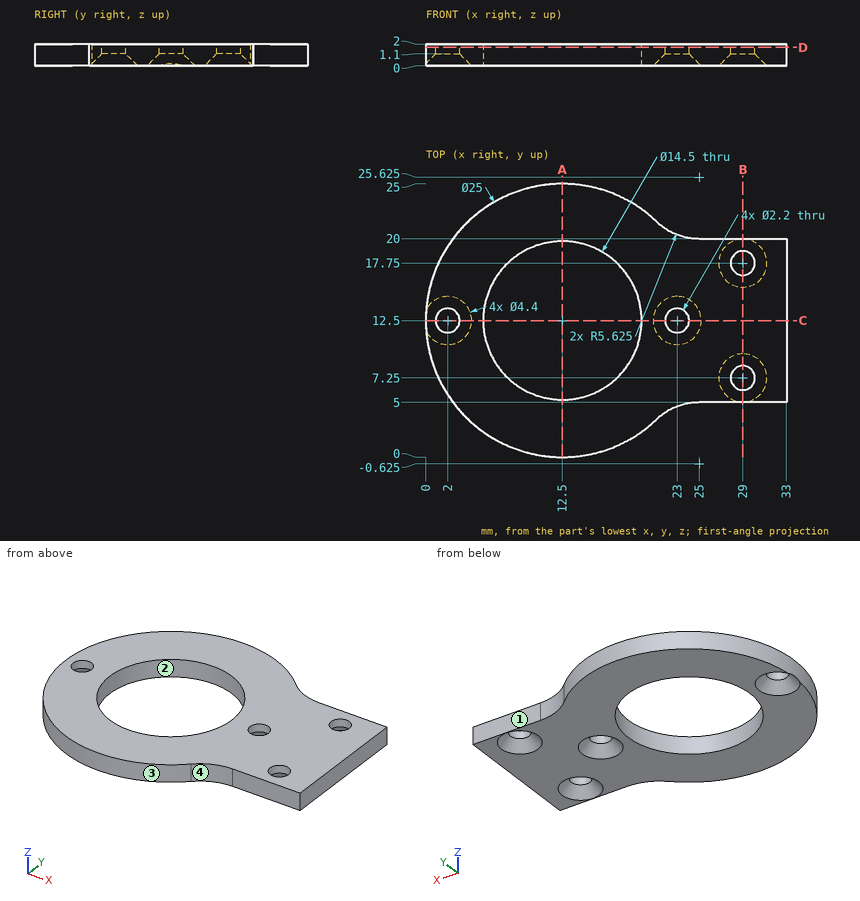
Geometry check sheet. Reference: drawing and pictorial views, mm from the part's lowest x, y, z. Round coordinates to 2 decimals unless told otherwise and drop trailing zeros. Order: outer loops, then holes, each group sorted by start corner. A loop starts at its lowest first (then second) coordinate and runs counter-clockwise, first axis right, second up. Notation, with made-up numbers: (20.5, 57.5) -> (49.5, 57.5) arc R36 ccw to (49.5, 92.5) -> close; hole circle Ø9 at (6, -2). An arc over 180 degrees is marked (long way). One line per item, written item: value. Start each with the question number.
Q1. Cross-section at C-C (y = 12.5). Record the boundary of the cut face in (x, z).
Q2. Gauge pin test, flat ends, axial feed: pin 1 Ø0.6 at (x, z) = (28.5, 1) entering from +Y; pin 2 Ø1.3 at (x, y) = (23, 12.5) entering from +Z; pin 3 Ø3.5 at (x, y) = (29, 7.25) entering from -Z. Record the tip position at first contact, or that the pin passes through.
Q3. Cross-section at A-A (x = 12.5). Record the boundary of the cut face in (y, z), and give its area (3 significant figures).
Q4. Cross-section at D-D (z = 1.7). Record the boundary of the cut face in (x, y) (3 decimals), and give its area (3 significant figures).
Q5. Mould release check, pull along Y, two halves, no side actions. Record for the marked faces 1, 2, 3 and 4: pulls with the +Y half, pulls with the -Y half, needs draft (parallel to the pull), parting line crosses it, or undercut.
Q6. Cross-section at B-B (x = 29). Record the boundary of the cut face in (y, z), and give its area (3 significant figures).
Q7. Thickness scan on line 1 (Y direction, x = 12.5, z = 1.4); line 2 (X direction, y = 18.5, z = 0.4); line 3 (X direction, y = 6.25, z = 1.7) (1 decimal). Record the ranges inside material, lowest first.
Completed:
1. outline: (0, 0.2) -> (0.9, 1.1) -> (0.9, 2) -> (0, 2) -> close; (3.1, 1.1) -> (4.2, 0) -> (5.25, 0) -> (5.25, 2) -> (3.1, 2) -> close; (19.75, 0) -> (20.8, 0) -> (21.9, 1.1) -> (21.9, 2) -> (19.75, 2) -> close; (24.1, 1.1) -> (25.2, 0) -> (33, 0) -> (33, 2) -> (24.1, 2) -> close
2. pin 1: stops at y = 20
2. pin 2: passes through
2. pin 3: stops at z = 0.45
3. outline: (0, 0) -> (5.25, 0) -> (5.25, 2) -> (0, 2) -> close; (19.75, 0) -> (25, 0) -> (25, 2) -> (19.75, 2) -> close
3. area: 21.0 mm²
4. outline: (21.121, 3.448) arc R5.625 cw to (25, 5) -> (33, 5) -> (33, 20) -> (25, 20) arc R5.625 cw to (21.121, 21.552) arc R12.5 ccw (long way) to start; hole circle Ø2.2 at (2, 12.5); hole circle Ø14.5 at (12.5, 12.5); hole circle Ø2.2 at (23, 12.5); hole circle Ø2.2 at (29, 7.25); hole circle Ø2.2 at (29, 17.75)
4. area: 444 mm²
5. face 1: pulls with the +Y half
5. face 2: undercut
5. face 3: parting line crosses it
5. face 4: pulls with the -Y half
6. outline: (5, 0) -> (5.05, 0) -> (6.15, 1.1) -> (6.15, 2) -> (5, 2) -> close; (8.35, 1.1) -> (9.45, 0) -> (15.55, 0) -> (16.65, 1.1) -> (16.65, 2) -> (8.35, 2) -> close; (18.85, 1.1) -> (19.95, 0) -> (20, 0) -> (20, 2) -> (18.85, 2) -> close
6. area: 18.8 mm²
7. line 1: y = 0 to 5.25, 19.75 to 25
7. line 2: x = 1.53 to 8.43, 16.57 to 27.36, 30.64 to 33
7. line 3: x = 1.7 to 8.8, 16.2 to 28.5, 29.5 to 33
